Geometry: final body of the model. Coordinates: model frame, mm. Round coordinates to 2 decimals unless told otherwise and drop trailing zeros. Loops run counter-clockwise (first coordinate to the right, second up) from the corner with the lowest first, then second, coordinate; pieces in that order, holes last. Notation, with made-up numbers: M 18.25,36.25 L 56.25,36.25 A26 ccw 56.25,70.25 Z; hole C 35.25,2.5 d8. An arc over 180 degrees is marked long. Answer as a JSON object with one key per item and string values.
```python
from build123d import *

# Parameters (mm, degrees)
BOSS_EXTRUDE2_DEPTH                          = 2
CHAMFER2_SIZE                                = 12
FILLET1_R                                    = 7.5
SKETCH2_R                                    = 2.575
SKETCH2_R_2                                  = 11.25
SKETCH2_R_3                                  = 3
CUT_EXTRUDE1_DEPTH                           = 290.359637821
CSK_FOR_M3_COUNTERSUNK_FLAT_HEAD_SCR_2_COUNT = 2
CSK_FOR_M3_COUNTERSUNK_FLAT_HEAD_SCR_2_PITCH = 31
CSK_FOR_M3_COUNTERSUNK_FLAT_HEAD_SCR_3_COUNT = 2
CSK_FOR_M3_COUNTERSUNK_FLAT_HEAD_SCR_3_PITCH = 43.840620434
CSK_FOR_M3_COUNTERSUNK_FLAT_HEAD_SCR_4_COUNT = 2
CSK_FOR_M3_COUNTERSUNK_FLAT_HEAD_SCR_4_PITCH = 31


with BuildPart() as part:
    # Sketch1 → Boss-Extrude2 (new body)
    with BuildSketch(Plane(origin=(0, 0, 0), x_dir=(1, 0, 0), z_dir=(0, 1, 0))):
        Polygon((40, -50), (77.320508076, -40), (285, -40), (285, 40), (77.320508076, 40), (40, 50), (-40, 50), (-122, 50), (-122, -50), (-40, -50), align=None)
    extrude(amount=BOSS_EXTRUDE2_DEPTH)

    # Chamfer2
    chamfer2_edges = [part.edges().sort_by_distance(p)[0] for p in [
        (-122, 1, 50),
        (-122, 1, -50),
        (285, 1, -40),
        (285, 1, 40),
    ]]
    chamfer(chamfer2_edges, length=CHAMFER2_SIZE)

    # Fillet1
    fillet1_edges = [part.edges().sort_by_distance(p)[0] for p in [
        (40, 1, -50),
        (77.320508076, 1, -40),
        (77.320508076, 1, 40),
        (40, 1, 50),
        (-110, 1, 50),
        (-122, 1, -38),
        (-122, 1, 38),
        (-110, 1, -50),
        (273, 1, -40),
        (285, 1, 28),
        (285, 1, -28),
        (273, 1, 40),
    ]]
    fillet(fillet1_edges, radius=FILLET1_R)

    # Sketch2 → Cut-Extrude1 (cut, through all)
    with BuildSketch(Plane(origin=(0, 2, 0), x_dir=(1, 0, 0), z_dir=(0, 1, 0))):
        with Locations(Location((-40, 40, 0), (0, 0, 270))):
            Circle(SKETCH2_R)
        with Locations(Location((40, 40, 0), (0, 0, 90))):
            Circle(SKETCH2_R)
        with Locations(Location((40, -40, 0), (0, 0, 270))):
            Circle(SKETCH2_R)
        with Locations(Location((-40, -40, 0), (0, 0, 90))):
            Circle(SKETCH2_R)
        with Locations(Location((-91, 0, 0), (0, 0, 270))):
            Circle(SKETCH2_R_2)
        with Locations(Location((0, 0, 0), (0, 0, 270))):
            Circle(SKETCH2_R_3)
    extrude(amount=-CUT_EXTRUDE1_DEPTH, mode=Mode.SUBTRACT)

    # Sketch4 → CSK for M3 Countersunk Flat Head Screw2 (revolve, cut)
    with BuildSketch(Plane(origin=(-106.5, 0, -15.5), x_dir=(0, 0, -1), z_dir=(1, 0, 0))):
        Polygon((0, 0), (0, 2), (1.7, 2), (1.7, 1.45), (3.15, 0), align=None)
    csk_for_m3_countersunk_flat_head_screw2 = revolve(axis=Axis((-106.5, -6.35, -15.5), (0, 1, 0)), mode=Mode.SUBTRACT)

    # CSK for M3 Countersunk Flat Head Scr 2: CSK for M3 Countersunk Flat Head Screw2 ×2
    with Locations(*[(0, 0, i * CSK_FOR_M3_COUNTERSUNK_FLAT_HEAD_SCR_2_PITCH) for i in range(1, CSK_FOR_M3_COUNTERSUNK_FLAT_HEAD_SCR_2_COUNT)]):
        add(csk_for_m3_countersunk_flat_head_screw2, mode=Mode.SUBTRACT)

    # CSK for M3 Countersunk Flat Head Scr 3: CSK for M3 Countersunk Flat Head Screw2 ×2
    with Locations(*[Vector(0.707106781186545, 0, 0.70710678118655) * (i * CSK_FOR_M3_COUNTERSUNK_FLAT_HEAD_SCR_3_PITCH) for i in range(1, CSK_FOR_M3_COUNTERSUNK_FLAT_HEAD_SCR_3_COUNT)]):
        add(csk_for_m3_countersunk_flat_head_screw2, mode=Mode.SUBTRACT)

    # CSK for M3 Countersunk Flat Head Scr 4: CSK for M3 Countersunk Flat Head Screw2 ×2
    with Locations(*[(i * CSK_FOR_M3_COUNTERSUNK_FLAT_HEAD_SCR_4_PITCH, 0, 0) for i in range(1, CSK_FOR_M3_COUNTERSUNK_FLAT_HEAD_SCR_4_COUNT)]):
        add(csk_for_m3_countersunk_flat_head_screw2, mode=Mode.SUBTRACT)


solid = part.part
```
1) Cut plane B-B on x = -91. Return the cut outline in (y, z), and give its area (3 significant figures).
Geometry results:
{"outline": "M 0,-50 L 2,-50 L 2,-11.25 L 0,-11.25 Z; M 0,11.25 L 2,11.25 L 2,50 L 0,50 Z", "area": "155 mm2"}
2) First-contact query: pin 1 (2.5 mm diameter, centred on x = -106.5, z = -15.5, fed in from -Y). Flat tip, straight axial feed; report the tip coordinate or a pass-through.
Geometry results:
{"pin 1": "through"}
3) Line query: probe 1 along X at (y, z) = (1.9, 15.5); probe 2 along X at (y, z) = (0.8, 0); probe 3 along Z at (x, y) = (-106.5, 1.9). Output: solid intervals per line, ascending.
Geometry results:
{"probe 1": "-122 to -108.2, -104.8 to -77.2, -73.8 to 285", "probe 2": "-122 to -102.25, -79.75 to -3, 3 to 285", "probe 3": "-50 to -17.2, -13.8 to 13.8, 17.2 to 50"}
4) Cut plane D-D on x = 53. Return the cut outline in (y, z), and give its area (3 significant figures).
Geometry results:
{"outline": "M 0,-46.52 L 2,-46.52 L 2,46.52 L 0,46.52 Z", "area": "186 mm2"}
5) Pull-direction query (X, two-part tool) for faces 1 (the face through (79, 0, -1)), 2 (the face through (-79.846, 1.014, -1.465)), 3 (the face through (279, 1, -34)); classes: +X half, -X half, draft (parallel to the pull), parting line (faces both ways), or undercut.
Geometry results:
{"face 1": "draft", "face 2": "undercut", "face 3": "+X half"}
6) Cut plane A-A on y = 0.45. Count the separate pieces of the cut face and the enclosed holes in it, and give its area (3 significant figures).
Geometry results:
{"separate pieces": "1", "enclosed holes": "10", "area": "35,300 mm2"}
7) Cut plane C-C on x = 205.5. Return the cut outline in (y, z).
Geometry results:
{"outline": "M 0,-40 L 2,-40 L 2,40 L 0,40 Z"}
